Could you check a few things on this model? Use its own coordinates, in mm. A direction names the side the tool comes from. Give positions to 0.01 mm unless a question says otherwise; leave off trailing zeros. Write each loop counter-clockwise with the first axis right and the second up, starting at its lowest first coordinate (ties: lowest second). Pieces come first, ordered by that corner, then holes. Notation, with made-up numbers: M -33,76.5 L -21,76.5 A18 ccw -21,98.5 Z; hole C 87,42 d7. An arc over 180 degrees is marked long. Answer as CSV lines item,"result". Start each with the question number.
Autodesk Fusion 360 part; units mm, degrees
sketch "Sketch1" plane through (0, 0, 0) normal (0, 0, 1) x (1, 0, 0)
  line L0 (0, 0) -> (0, 92.3036)
  line L1 (0, 0) -> (71.9074, 0)
  line L2 (71.9074, 0) -> (71.9074, 92.3036)
  line L3 (71.9074, 92.3036) -> (0, 92.3036)
  line L4 (5, 5) -> (66.9074, 5)
  line L5 (66.9074, 5) -> (66.9074, 87.3036)
  line L6 (66.9074, 87.3036) -> (5, 87.3036)
  line L7 (5, 5) -> (5, 87.3036)
  dimension "d1" = 92.3036
  dimension "d2" = 71.9074
  dimension "d3" = 5
extrude "Extrude1" add sketch "Sketch1" against normal blind 3 contours L0 L1 L2 L3 | L4 L5 L6 L7
extrude "Extrude2" add sketch "Sketch1" along normal blind 10
fillet "Fillet1" radius 2 4 edges at (71.9074, 0, 3.5) (0, 0, 3.5) (0, 92.3036, 3.5) (71.9074, 92.3036, 3.5)
sketch "Sketch2" plane through (0, 0, 10) normal (0, 0, 1) x (-1, 0, 0)
  line L0 (-66.9074, -87.3036) -> (-66.9074, -5)
  line L1 (-66.9074, -5) -> (-5, -5)
  line L2 (-5, -5) -> (-5, -87.3036)
  line L3 (-5, -87.3036) -> (-66.9074, -87.3036)
  arc A0 (-71.9074, -90.3036) -> (-69.9074, -92.3036) centre (-69.9074, -90.3036) ccw
  line L4 (-69.9074, -92.3036) -> (-2, -92.3036)
  arc A1 (-2, -92.3036) -> (0, -90.3036) centre (-2, -90.3036) ccw
  line L5 (0, -90.3036) -> (0, -2)
  arc A2 (0, -2) -> (-2, 0) centre (-2, -2) ccw
  line L6 (-2, 0) -> (-69.9074, 0)
  arc A3 (-69.9074, 0) -> (-71.9074, -2) centre (-69.9074, -2) ccw
  line L7 (-71.9074, -2) -> (-71.9074, -90.3036)
  circle A4 centre (-68.4022, -3.5052) radius 1.7145
  line L8 (-35.9537, -92.3036) -> (-35.9537, 0)
  circle A5 centre (-3.5052, -3.5052) radius 1.7145
  line L9 (-67.4347, -46.1518) -> (-71.9074, -46.1518)
  line L10 (-67.4347, -46.1518) -> (0, -46.1518)
  circle A6 centre (-68.4022, -88.7984) radius 1.7145
  circle A7 centre (-3.5052, -88.7984) radius 1.7145
  dimension "d12" = 3.429
extrude "Extrude3" cut sketch "Sketch2" against normal blind 5 contours A4 | A5 | A6 | A7
1. Please list where these lines run through material, in increasing order: line 1 (X direction, y = 28, z = 8.5); line 2 (Y direction, x = 22.5, z = 6.5); line 3 (Y direction, x = 3.5, z = 6.75).
2. Imagine slicing it at D-D, the plane z = 8.5. Please give me the cut outline in (x, y), plus the area to 3 significant figures.
3. On a 3-axis mill with a long thin cutter (end or side, diameter ignored), from which of +Z, -Z, +X, -X, +Y, -Y can I reach the whole of each face in a straight line? I mean faces 1 (the flat face through (36, 87.304, 5)), 2 (the cylindrical face through (71.306, 0.57, 3.591)). Say none if no direction works.
4. Imagine slicing it at B-B, the plane z = 3. Please give me the cut outline in (x, y), plus the area to 3 significant figures.
5. Imagine slicing it at C-C, the plane y = 77.5. Please give me the cut outline in (x, z).
6. Thinking about a two-plate mould opening in X: for faces 3 (the flat face through (68, 89, 5)), 4 (the cylindrical face through (71.31, 91.73, 3.41)), 5 (the cylindrical face through (0.57, 91.7, 3.41)), which applies, pulls with the +X half, pulls with the -X half, needs draft (parallel to the pull), parting line crosses it, or undercut?
7. Will these pins go through, and if not, where does the flat tip stop? P1, Ø2.5, axis at x = 68.5, y = 3.5, coming from the +Z side; P2, Ø10, axis at x = 39.5, y = 37, coming from the +Z side.
8. Imagine slicing it at A-A, the plane x = 36.5. Please give me the cut outline in (y, z), plus the area to 3 significant figures.
Solutions:
1,line 1,"0 to 5, 66.91 to 71.91"
1,line 2,"0 to 5, 87.3 to 92.3"
1,line 3,"0 to 1.79, 5.22 to 87.08, 90.51 to 92.3"
2,outline,"M 0,2 A2 ccw 2,0 L 69.91,0 A2 ccw 71.91,2 L 71.91,90.3 A2 ccw 69.91,92.3 L 2,92.3 A2 ccw 0,90.3 Z; hole C 3.51,3.51 d3.43; hole C 3.51,88.8 d3.43; hole M 5,5 L 66.91,5 L 66.91,87.3 L 5,87.3 Z; hole C 68.4,3.51 d3.43; hole C 68.4,88.8 d3.43"
2,area,"1,500 mm²"
3,face 1,"+Z"
3,face 2,"+Z, -Z, +X, -Y"
4,outline,"M 0,2 A2 ccw 2,0 L 69.91,0 A2 ccw 71.91,2 L 71.91,90.3 A2 ccw 69.91,92.3 L 2,92.3 A2 ccw 0,90.3 Z; hole M 5,5 L 66.91,5 L 66.91,87.3 L 5,87.3 Z"
4,area,"1,540 mm²"
5,outline,"M 0,-3 L 71.91,-3 L 71.91,10 L 66.91,10 L 66.91,0 L 5,0 L 5,10 L 0,10 Z"
6,face 3,"undercut"
6,face 4,"pulls with the +X half"
6,face 5,"pulls with the -X half"
7,P1,"z = 5"
7,P2,"z = 0"
8,outline,"M 0,-3 L 92.3,-3 L 92.3,10 L 87.3,10 L 87.3,0 L 5,0 L 5,10 L 0,10 Z"
8,area,"377 mm²"
